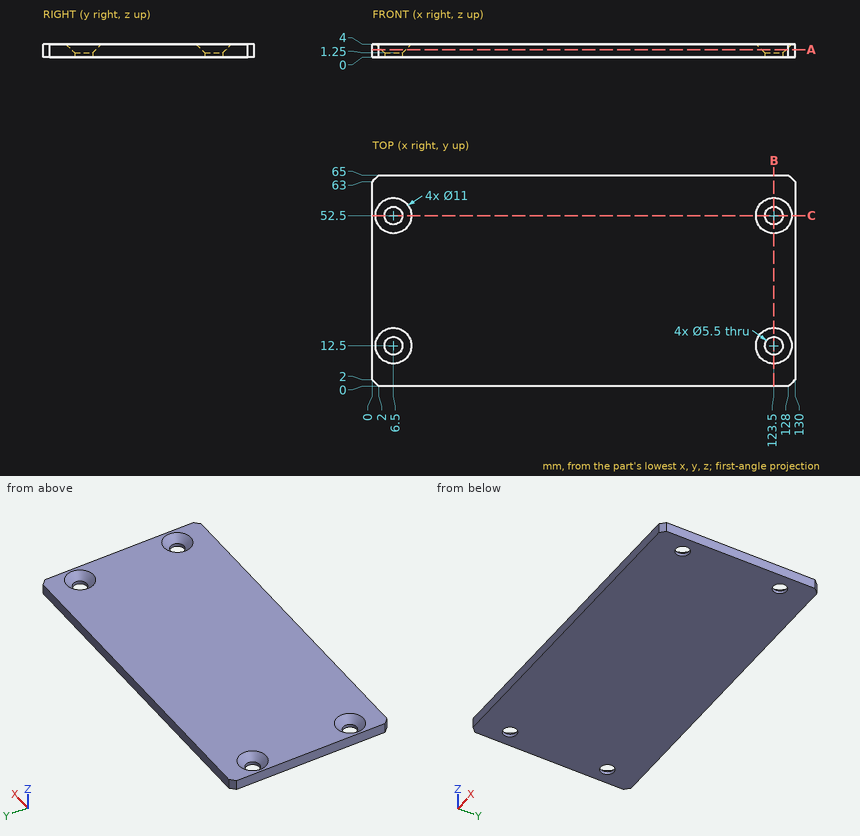
Source: three-view drawing plus pictorial views. Frame: mm from the lowest corner of the part. Give positions to 0.01 mm unless a question says otherwise; leave off trailing zeros. Order: outer loops, then holes, each group sorted by start corner. A loop starts at its lowest first (then second) coordinate and runs counter-clockwise, first axis right, second up. Notation, with made-up numbers: (-23.75, 46) -> (17.25, 46) arc R23 cw to (17.25, 76) -> close; hole circle Ø9 at (48, -11). An arc over 180 degrees is marked (long way). Write each question's results on one line, items separated by ' | '. Start each with the question number.
Item 1: Contact query for flat-ended pins moving along their axis: P1, Ø4.5, axis at x = 6.5, y = 12.5, coming from the -Z side; P2, Ø7, axis at x = 6.5, y = 52.5, coming from the +Z side. Output: stop coordinate, or through.
Item 2: Cut plane A-A on z = 2.3. Return the cut outline in (x, y), then the cut area to 3 significant figures.
Item 3: Line query: line 1 (X direction, y = 12.5, z = 0.6); line 2 (Y direction, x = 123.5, z = 0.75); line 3 (Z direction, x = 6, y = 17). Output: solid intervals per line, ascending.
Item 4: Cut plane C-C on y = 52.5. Return the cut outline in (x, z).
Item 5: Cut plane B-B on x = 123.5. Return the cut outline in (y, z), then the cut area to 3 significant figures.
Established:
1) P1: through | P2: z = 2
2) outline: (0, 2) -> (2, 0) -> (128, 0) -> (130, 2) -> (130, 63) -> (128, 65) -> (2, 65) -> (0, 63) -> close; hole circle Ø7.6 at (6.5, 12.5); hole circle Ø7.6 at (6.5, 52.5); hole circle Ø7.6 at (123.5, 12.5); hole circle Ø7.6 at (123.5, 52.5) | area: 8,260 mm^2
3) line 1: 0 to 3.75, 9.25 to 120.75, 126.25 to 130 | line 2: 0 to 9.75, 15.25 to 49.75, 55.25 to 65 | line 3: 0 to 3.03
4) outline: (0, 0) -> (3.75, 0) -> (3.75, 1.25) -> (1, 4) -> (0, 4) -> close; (9.25, 0) -> (120.75, 0) -> (120.75, 1.25) -> (118, 4) -> (12, 4) -> (9.25, 1.25) -> close; (126.25, 0) -> (130, 0) -> (130, 4) -> (129, 4) -> (126.25, 1.25) -> close
5) outline: (0, 0) -> (9.75, 0) -> (9.75, 1.25) -> (7, 4) -> (0, 4) -> close; (15.25, 0) -> (49.75, 0) -> (49.75, 1.25) -> (47, 4) -> (18, 4) -> (15.25, 1.25) -> close; (55.25, 0) -> (65, 0) -> (65, 4) -> (58, 4) -> (55.25, 1.25) -> close | area: 201 mm^2
